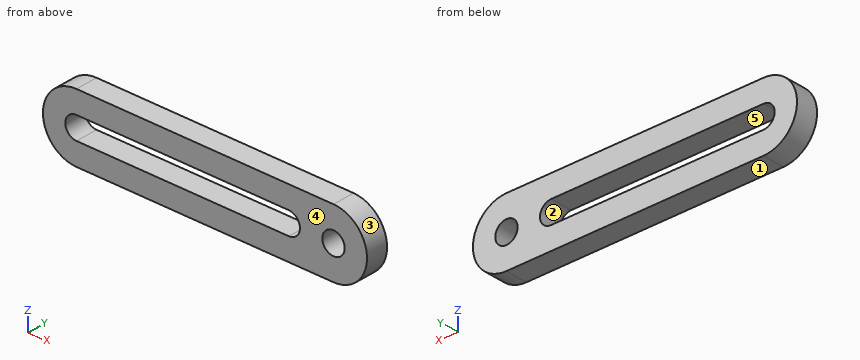
```python
from build123d import *

# Parameters (mm, degrees)
SKETCH1_R           = 5
BOSS_EXTRUDE1_DEPTH = 10


with BuildPart() as part:
    # Sketch1 → Boss-Extrude1 (new body)
    with BuildSketch(Plane(origin=(0, 0, 0), x_dir=(1, 0, 0), z_dir=(0, 1, 0))):
        with BuildLine():
            Line((0, 15), (115, 15))
            ThreePointArc((115, 15), (130, 0), (115, -15))
            Line((115, -15), (0, -15))
            ThreePointArc((0, -15), (-15, 0), (0, 15))
        make_face()
        with Locations((115, 0)):
            Circle(SKETCH1_R, mode=Mode.SUBTRACT)
        with BuildLine():
            Line((0, 5), (95, 5))
            ThreePointArc((95, 5), (100, 0), (95, -5))
            Line((95, -5), (0, -5))
            ThreePointArc((0, -5), (-5, 0), (0, 5))
        make_face(mode=Mode.SUBTRACT)
    extrude(amount=BOSS_EXTRUDE1_DEPTH)


solid = part.part
```
Design review of the part built by this model. Coordinates are the model's own, in mm. Face numbers are marked on the shaded views. A direction names the side the tool comes from. Give positions to 0.01 mm unless a question says otherwise; leave off trailing zeros. Order: outer loops, then holes, each group sorted by start corner. A loop starts at its lowest first (then second) coordinate and runs counter-clockwise, first axis right, second up. Notation, with made-up numbers: (-11, 83.25) - (-4, 83.25) arc R10 cw to (-4, 102.25) - close; hole circle Ø2 at (-25.5, 87.25). An arc over 180 degrees is marked (long way). Use a Markdown table: item, result. Add a question column.
(1) Add section B-B on y = 3.25. Give the boundary of the cut face in (x, z).
(2) Add section D-D on z = 10. Give the boundary of the cut face in (x, y).
(3) Machinability: for the marked faces 1 and 2, which of the approach directions +Z, -Z, +X, -X, +Y, -Y give a long, thin tool a straight path to every point of the face, cutting with its end or side? Answer none if there is none.
(4) Mouldability with a two-part tool opening along Z and no side actions: class the marked faces 3, 4 and 5 as +Z half, -Z half, draft (parallel to the pull), parting line (faces both ways), or undercut.
(5) Add section A-A on z = 0. Give the boundary of the cut face in (x, y).
(6) Clearance check with flat-ended pins moving along their axes: P1, Ø8, axis at x = 115, z = 0, coming from the +Y side; P2, Ø6, axis at y = 8.5, z = 4.5, coming from the +X side; P3, Ø6, axis at y = 1.5, z = 8.5, coming from the -X side. State where each tip first meets the part, or that it passes through.
(7) Add section C-C on x = 24. Give the boundary of the cut face in (y, z), then the cut area to 3 significant figures.
(8) Wall thickness on probe 1 along X at (y, z) = (5.25, 0); probe 2 along Z at (x, y) = (34, 6.5); probe 3 along X at (y, z) = (9, -4): over which ranges is each line inside the solid? List them lowest first. Write a range as [from, to].
Report:
| question | item | result |
|---|---|---|
| 1 | outline | (0, -15) - (115, -15) arc R15 ccw to (115, 15) - (0, 15) arc R15 ccw to start; hole (0, -5) - (95, -5) arc R5 ccw to (95, 5) - (0, 5) arc R5 ccw to start; hole circle Ø10 at (115, 0) |
| 2 | outline | (-11.18, 0) - (126.18, 0) - (126.18, 10) - (-11.18, 10) - close |
| 3 | face 1 | -Z, +X, -X, +Y, -Y |
| 3 | face 2 | +Y, -Y |
| 4 | face 3 | parting line |
| 4 | face 4 | draft |
| 4 | face 5 | undercut |
| 5 | outline | (-15, 0) - (-5, 0) - (-5, 10) - (-15, 10) - close; (100, 0) - (110, 0) - (110, 10) - (100, 10) - close; (120, 0) - (130, 0) - (130, 10) - (120, 10) - close |
| 6 | P1 | passes through |
| 6 | P2 | stops at x = 129.92 |
| 6 | P3 | stops at x = -13.96 |
| 7 | outline | (0, -15) - (10, -15) - (10, -5) - (0, -5) - close; (0, 5) - (10, 5) - (10, 15) - (0, 15) - close |
| 7 | area | 200 mm² |
| 8 | probe 1 | x = [-15, -5], [100, 110], [120, 130] |
| 8 | probe 2 | z = [-15, -5], [5, 15] |
| 8 | probe 3 | x = [-14.46, -3], [98, 112], [118, 129.46] |
